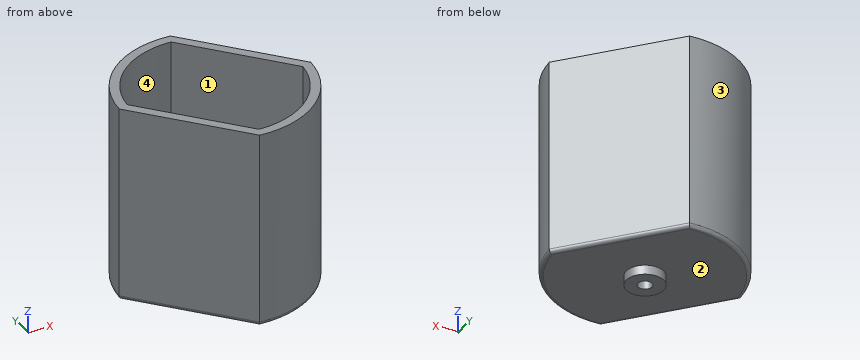
from build123d import *

# Parameters (mm, degrees)
BOSS_EXTRUDE1_DEPTH = 20
BOSS_EXTRUDE2_START = 1
BOSS_EXTRUDE2_DEPTH = 1
FILLET1_R           = 0.4
SKETCH3_R           = 2
BOSS_EXTRUDE3_DEPTH = 1
SKETCH4_R           = 0.75
CUT_EXTRUDE1_DEPTH  = 27.150121814


with BuildPart() as part:
    # Sketch1 → Boss-Extrude1 (new body)
    with BuildSketch(Plane.XY):
        with BuildLine():
            Line((-9.991439682, 0.413682349), (-0.473124093, -9.988801409))
            ThreePointArc((-0.473124093, -9.988801409), (6.750578432, -7.377648056), (9.991439682, -0.413682349))
            Line((9.991439682, -0.413682349), (0.473124093, 9.988801409))
            ThreePointArc((0.473124093, 9.988801409), (-6.750578432, 7.377648056), (-9.991439682, 0.413682349))
        make_face()
        with BuildLine():
            Line((-8.966572571, 0.774968597), (-0.022461592, -8.999971971))
            ThreePointArc((-0.022461592, -8.999971971), (6.075520589, -6.63988325), (8.966572571, -0.774968597))
            Line((8.966572571, -0.774968597), (0.022461592, 8.999971971))
            ThreePointArc((0.022461592, 8.999971971), (-6.075520589, 6.63988325), (-8.966572571, 0.774968597))
        make_face(mode=Mode.SUBTRACT)
    extrude(amount=BOSS_EXTRUDE1_DEPTH)

    # Sketch2 → Boss-Extrude2 (add)
    with BuildSketch(Plane(origin=(0, 0, 0), x_dir=(-1, 0, 0), z_dir=(0, 0, -1)).offset(BOSS_EXTRUDE2_START)):
        with BuildLine():
            Line((-0.473124093, 9.988801409), (-9.991439682, -0.413682349))
            ThreePointArc((-9.991439682, -0.413682349), (-6.750578432, -7.377648056), (0.473124093, -9.988801409))
            Line((0.473124093, -9.988801409), (9.991439682, 0.413682349))
            ThreePointArc((9.991439682, 0.413682349), (6.750578432, 7.377648056), (-0.473124093, 9.988801409))
        make_face()
    extrude(amount=-BOSS_EXTRUDE2_DEPTH)

    # Fillet1
    fillet1_edges = [part.edges().sort_by_distance(p)[0] for p in [
        (-6.750578432, 7.377648056, -1),
        (5.232281887, 4.78755953, -1),
        (6.750578432, -7.377648056, -1),
        (-5.232281887, -4.78755953, -1),
    ]]
    fillet(fillet1_edges, radius=FILLET1_R)

    # Sketch3 → Boss-Extrude3 (add)
    with BuildSketch(Plane(origin=(0, 0, -1), x_dir=(-1, 0, 0), z_dir=(0, 0, -1))):
        Circle(SKETCH3_R)
    extrude(amount=BOSS_EXTRUDE3_DEPTH)

    # Sketch4 → Cut-Extrude1 (cut, through all)
    with BuildSketch(Plane(origin=(0, 0, -2), x_dir=(-1, 0, 0), z_dir=(0, 0, -1))):
        Circle(SKETCH4_R)
    extrude(amount=-CUT_EXTRUDE1_DEPTH, mode=Mode.SUBTRACT)


solid = part.part
Input: part model. Units: mm. Frame: model coordinates. Face numbers are marked on the shaded views. Give positions to 0.01 mm unless a question says otherwise; leave off trailing zeros. Write each loop counter-clockwise with the first axis right and the second up, starting at its lowest first coordinate (ties: lowest second). Pieces come first, ordered by that corner, then holes.
Q1. Material intervals for probe 1 along Y at (x, z) = (0, -1.3); probe 2 along Y at (x, z) = (0, -0.6); probe 3 along Z at (x, y) = (6.75, -0.75), sorted ascending.
Q2. First-contact query: P1, Ø1.5, axis at x = 3, y = 8, coming from the -Z side; P2, Ø5, axis at x = -3.5, z = 11.5, coming from the +Y side; P3, Ø2, axis at x = -8, z = 1, coming from the +Y side; P4, Ø8, axis at x = -1.5, y = -3, coming from the -Z side. Flat tips, straight axial feed; report the tip coordinate or a pass-through.
Q3. Section A-A, the plane z = 12. Output: boundary loops of the cut face in (x, y), plus the area to 3 significant figures.
Q4. Pull-direction query (Y, two-part tool) for the marked faces 1, 2, 3 and 4; classes: pulls with the +Y half, pulls with the -Y half, needs draft (parallel to the pull), parting line crosses it, or undercut.
Filled in:
1. probe 1: y = -2 to -0.75, 0.75 to 2
1. probe 2: y = -10 to -0.75, 0.75 to 10
1. probe 3: z = -1 to 0
2. P1: stops at z = -0.96
2. P2: stops at y = 9.95
2. P3: stops at y = 7.14
2. P4: stops at z = -2
3. outline: (-9.99, 0.41) - (-0.47, -9.99) arc R10 ccw to (9.99, -0.41) - (0.47, 9.99) arc R10 ccw to start; hole (-8.97, 0.77) - (-0.02, -9) arc R9 ccw to (8.97, -0.77) - (0.02, 9) arc R9 ccw to start
3. area: 56.5 mm2
4. face 1: undercut
4. face 2: needs draft
4. face 3: pulls with the +Y half
4. face 4: undercut
